```python
from build123d import *

# Parameters (mm, degrees)
SKETCH_1_R      = 1.5
EXTRUDE_1_DEPTH = 30
SKETCH_2_R      = 2
SKETCH_2_R_2    = 1.5
EXTRUDE_2_DEPTH = 14.5
FILLET_1_R      = 0.1
SKETCH_3_R      = 2.5
SKETCH_3_R_2    = 2
EXTRUDE_3_DEPTH = 0.5


with BuildPart() as part:
    # 草图1 → 凸台-拉伸1 (new body)
    with BuildSketch(Plane(origin=(0, 0, 0), x_dir=(1, 0, 0), z_dir=(0, 1, 0))):
        with Locations(Location((0, 0, 0), (0, 0, 270))):
            Circle(SKETCH_1_R)
    extrude(amount=EXTRUDE_1_DEPTH)

    # 草图2 → 凸台-拉伸2 (add)
    with BuildSketch(Plane(origin=(0, 12, 0), x_dir=(1, 0, 0), z_dir=(0, 1, 0))):
        with Locations(Location((0, 0, 0), (0, 0, 90))):
            Circle(SKETCH_2_R)
        with Locations(Location((0, 0, 0), (0, 0, 270))):
            Circle(SKETCH_2_R_2, mode=Mode.SUBTRACT)
    extrude(amount=EXTRUDE_2_DEPTH)

    # 圆角1
    fillet_1_edges = [part.edges().sort_by_distance(p)[0] for p in [
        (0, 0, -1.5),
        (0, 30, -1.5),
    ]]
    fillet(fillet_1_edges, radius=FILLET_1_R)

    # 草图3 → 凸台-拉伸3 (add)
    with BuildSketch(Plane(origin=(0, 12, 0), x_dir=(-1, 0, 0), z_dir=(0, -1, 0))):
        with Locations(Location((0, 0, 0), (0, 0, 90))):
            Circle(SKETCH_3_R)
        with Locations(Location((0, 0, 0), (0, 0, 90))):
            Circle(SKETCH_3_R_2, mode=Mode.SUBTRACT)
    extrude(amount=-EXTRUDE_3_DEPTH)


solid = part.part
```
Could you check a few things on this model? Use its own coordinates, in mm. A direction names the side the tool comes from. Give positions to 0.01 mm unless a question says otherwise; leave off trailing zeros. Loops run counter-clockwise (first coordinate to the right, second up) from the corner with the lowest first, then second, coordinate; pieces in that order, holes last. Notation, with made-up numbers: (59.5, -31) - (68.5, -31) arc R13 ccw to (68.5, -17) - close; hole circle Ø2 at (73, 61.5). An arc over 180 degrees is marked (long way). Answer in a Markdown table with one row per item. Add a question column.
Q1. Which directions (+Z, -Z, +X, -X, +Y, -Y) give clear straight access to the entire face, cutting with the end or side of a thin tool? Please do faces 1 (the face through (-2.44, 12.25, 0.54)), 2 (the face through (-2, 12, 0)), 3 (the face through (2, 19, 0)).
Q2. If we section it at A-A (z = 0): List the corners of the cut face in (x, y) for me, plus the area to 3 significant figures.
Q3. Please list where these lines run through material, in increasing order: L1, parallel to Y at x = -0.35, z = 2; L2, parallel to X at y = 5.5, z = 0.05; L3, parallel to X at y = 22.75, z = 0.1. Write a range as from..to.
Q4. If we section it at C-C (y = 16.25): List the corners of the cut face in (x, z) for me.
Q5. If we section it at B-B (x = 0): List the corners of the cut face in (y, z) for me.
Q6. If we section it at D-D (y = 11.5): List the corners of the cut face in (x, z) for me, plus the area to 3 significant figures.
Q7. For pin 1 (1 mm diameter, centred on y = 25.5, z = -1, fed in from +X); pin 2 (1.5 mm diameter, centred on x = -0.5, z = -0.5, fed in from -Y); pin 3 (1.5 mm diameter, centred on y = 6, z = -2, fed in from -X); pin 4 (1 mm diameter, centred on y = 24, z = 0, fed in from +X), each with a flat end and sliding along its axis, tell me the tip position at first contact or that it passes through.
The answers:
| question | item | result |
|---|---|---|
| 1 | face 1 | +Y, -Y |
| 1 | face 2 | -Y |
| 1 | face 3 | +Y |
| 2 | outline | (-2.5, 12) - (-1.5, 12) - (-1.5, 0.1) arc R0.1 ccw to (-1.4, 0) - (1.4, 0) arc R0.1 ccw to (1.5, 0.1) - (1.5, 12) - (2.5, 12) - (2.5, 12.5) - (2, 12.5) - (2, 26.5) - (1.5, 26.5) - (1.5, 29.9) arc R0.1 ccw to (1.4, 30) - (-1.4, 30) arc R0.1 ccw to (-1.5, 29.9) - (-1.5, 26.5) - (-2, 26.5) - (-2, 12.5) - (-2.5, 12.5) - close |
| 2 | area | 105 mm^2 |
| 3 | L1 | y = 12..12.5 |
| 3 | L2 | x = -1.5..1.5 |
| 3 | L3 | x = -2..2 |
| 4 | outline | circle Ø4 at (0, 0) |
| 5 | outline | (0, -1.4) arc R0.1 ccw to (0.1, -1.5) - (12, -1.5) - (12, -2.5) - (12.5, -2.5) - (12.5, -2) - (26.5, -2) - (26.5, -1.5) - (29.9, -1.5) arc R0.1 ccw to (30, -1.4) - (30, 1.4) arc R0.1 ccw to (29.9, 1.5) - (26.5, 1.5) - (26.5, 2) - (12.5, 2) - (12.5, 2.5) - (12, 2.5) - (12, 1.5) - (0.1, 1.5) arc R0.1 ccw to (0, 1.4) - close |
| 6 | outline | circle Ø3 at (0, 0) |
| 6 | area | 7.07 mm^2 |
| 7 | pin 1 | stops at x = 1.94 |
| 7 | pin 2 | stops at y = 0 |
| 7 | pin 3 | stops at x = -0.83 |
| 7 | pin 4 | stops at x = 2 |
